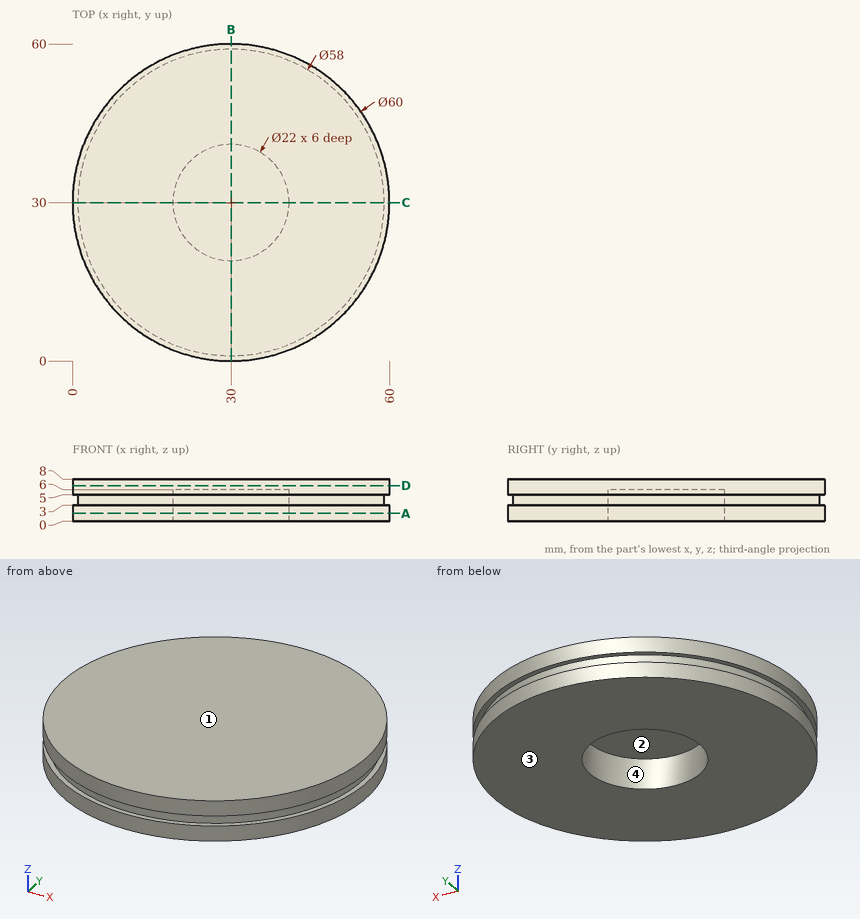
Can you work these out from the drawing? Everything is in mm from the part's minimum corner. A direction names the side the tool comes from. Round coordinates to 2 decimals unless told otherwise and drop trailing zeros. Loops run counter-clockwise (first coordinate to the right, second up) from the corner with the lowest first, then second, coordinate; pieces in that order, holes last. Notation, with made-up numbers: M 28,66.5 L 37,66.5 A6 cw 37,75.5 Z; hole C 42,67 d2. An arc over 180 degrees is marked long. Write item = value, one per line.
1. Will these pins go through, and if not, where does the flat tip stop? P1, Ø3, axis at y = 21.5, z = 4.5, coming from the +X side; P2, Ø4, axis at y = 25, z = 6.5, coming from the -X side.
Results below:
P1 = 59.15
P2 = 0.15
2. Thinking about a two-plate mould opening in Y: for the marked faces 3 and 4, which applies, +Y half, -Y half, draft (parallel to the pull), parting line (faces both ways), or undercut?
Results below:
face_3 = draft
face_4 = undercut
3. I want a section at B-B, the plane x = 30. Write out the boundary of the cut face in (y, z).
Results below:
outline = M 0,0 L 19,0 L 19,6 L 41,6 L 41,0 L 60,0 L 60,3 L 59,3 L 59,5 L 60,5 L 60,8 L 0,8 L 0,5 L 1,5 L 1,3 L 0,3 Z
4. Which directions (+Z, -Z, +X, -X, +Y, -Y) give clear straight access to the entire face, cutting with the end or side of a thin tool? Please do the marked faces 1 and 2.
Results below:
face_1 = +Z, +X, -X, +Y, -Y
face_2 = -Z
5. I need wall thicknesses on probe 1 along Y at (x, z) = (30, 1.3); probe 2 along Z at (x, y) = (55.5, 45); probe 3 along X at (y, z) = (35, 1). Which ranges of each line are inside material? Lowest first, please.
Results below:
probe_1 = 0 to 19, 41 to 60
probe_2 = 0 to 3, 5 to 8
probe_3 = 0.42 to 20.2, 39.8 to 59.58
6. I want a section at D-D, the plane z = 6.75. Write out the boundary of the cut face in (x, y).
Results below:
outline = C 30,30 d60
7. I want a section at A-A, the plane z = 1.5. Write out the boundary of the cut face in (x, y), and give its area (3 significant figures).
Results below:
outline = C 30,30 d60; hole C 30,30 d22
area = 2,450 mm²
